Can you work these out from the model? Positions are in its coordinate system, mm. Give positions to 0.01 mm unless a question says otherwise; leave off trailing zeros. Write each loop counter-clockwise with the first axis right and the second up, starting at its lowest first coordinate (ties: lowest second). Pieces come first, ordered by that corner, then holes.
Solid Edge part; units mm, degrees
sketch "Sketch1" plane through (0, 0, 0) normal (0, 0, 1) x (1, 0, 0)
  line L0 (-125, -20) -> (125, -20)
  line L1 (125, -20) -> (125, 20)
  line L2 (125, 20) -> (-125, 20)
  line L3 (-125, 20) -> (-125, -20)
extrude "Protrusion1" add sketch "Sketch1" against normal blind 32
sketch "Sketch2" plane through (0, -20, -16) normal (0, -1, 0) x (1, 0, 0)
  line L0 (-125, 16) -> (-60, 16)
  line L1 (-60, 16) -> (-125, 2.7756)
  line L2 (-125, 2.7756) -> (-125, 16)
extrude "ExtrudedCutout_1" cut sketch "Sketch2" against normal blind 180
fillet "Round_1" radius 20 1 edges at (-125, 0, -13.2244)
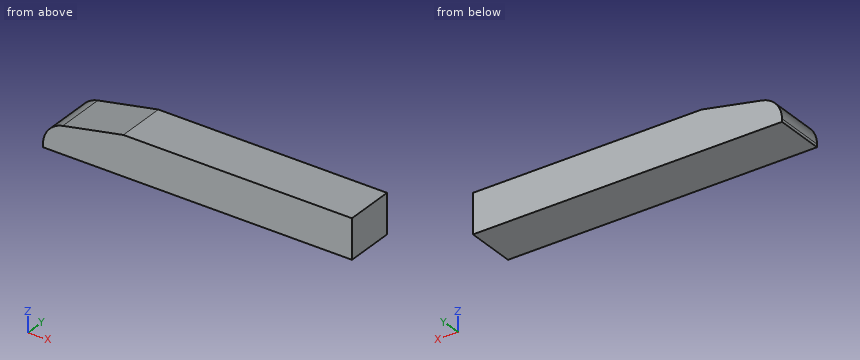
1) For pin 1 Ø4 at (y, z) = (4, -22.5) entering from -X; pin 2 Ø1 at (x, y) = (-68, 12.5) entering from +Z, each with a flat end and sliding along its axis, tell me the tip position at first contact or that it passes through.
Values follow:
pin 1: stops at x = -124.35
pin 2: stops at z = -1.53
2) Suppose I cut it at A-A on y = 0. Write out the boundary of the cut face in (x, z).
Values follow:
outline: (-125, -32) - (125, -32) - (125, 0) - (-60, 0) - (-108.99, -9.97) arc R20 ccw to (-125, -29.57) - close
3) Suppose I cut it at B-B on z = -5. Write out the boundary of the cut face in (x, y), plus the area to 3 significant figures.
Values follow:
outline: (-84.58, -20) - (125, -20) - (125, 20) - (-84.58, 20) - close
area: 8,380 mm2
4) Suppose I cut it at C-C on x = -72. Write out the boundary of the cut face in (y, z).
Values follow:
outline: (-20, -32) - (20, -32) - (20, -2.44) - (-20, -2.44) - close
5) Please list where these lines run through material, in increasing order: L1, parallel to X at y = 12, z = -14.5; L2, parallel to X at y = -5, z = -25.5; L3, parallel to Z at x = -65, y = -11.
Values follow:
L1: x = -118.15 to 125
L2: x = -124.58 to 125
L3: z = -32 to -1.02
